Design review of the part built by this model. Coordinates are the model's own, in mm. Face numbers are marked on the shaded views. A direction names the side the tool comes from. Give positions to 0.01 mm unless a question says otherwise; leave off trailing zeros. Order: outer loops, then holes, each group sorted by start corner. A loop starts at its lowest first (then second) coordinate and runs counter-clockwise, first axis right, second up.
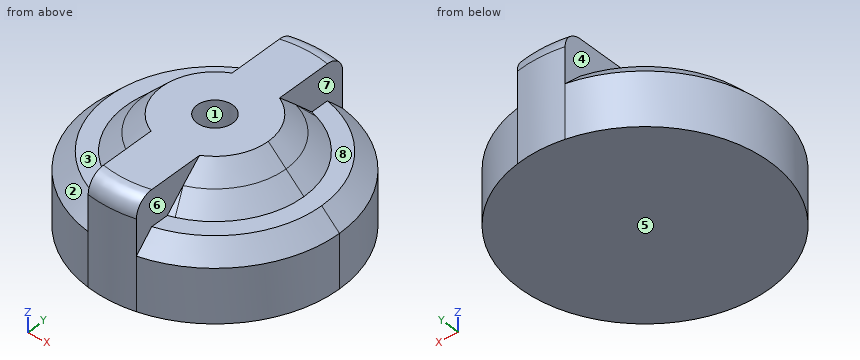
```python
from build123d import *
from build123d import SkipClean  # not in build123d's __all__

# Parameters (mm, degrees)
F0_R     = 3.175
F1_DEPTH = 12.7
F2_DEPTH = 19.05
F3_SIZE  = 3.17499
F4_DEPTH = 19.05
F5_R     = 3.175
F6_START = 6
F6_DEPTH = 15


# Not quite as in the source:
# - a fillet or chamfer is up to 0.001 mm smaller than in the source, because OpenCascade refuses the exact size


with BuildPart() as f1:
    # F0 (on Top) → F1 (new body)
    with BuildSketch(Plane.XY):
        with BuildLine():
            Line((-4.1830006975, 11.9913512652), (-4.1830006975, 21.8278063526))
            ThreePointArc((-4.1830006975, 21.8278063526), (-22.225, 0), (-4.1830006975, -21.8278063526))
            Line((-4.1830006975, -21.8278063526), (-4.1830006975, -11.9913512652))
            ThreePointArc((-4.1830006975, -11.9913512652), (-12.7, 0), (-4.1830006975, 11.9913512652))
        make_face()
        with BuildLine():
            ThreePointArc((4.3927960263, -21.7865547545), (17.1985539608, -14.0769445072), (22.225, 0))
            ThreePointArc((22.225, 0), (17.1985539608, 14.0769445072), (4.3927960263, 21.7865547545))
            Line((4.3927960263, 21.7865547545), (4.3927960263, 11.916095966))
            ThreePointArc((4.3927960263, 11.916095966), (10.4182174467, 7.2629708269), (12.7, 0))
            ThreePointArc((12.7, 0), (10.4182174467, -7.2629708269), (4.3927960263, -11.916095966))
            Line((4.3927960263, -11.916095966), (4.3927960263, -21.7865547545))
        make_face()
        with BuildLine():
            Line((4.3927960263, -11.916095966), (4.3927960263, 11.916095966))
            ThreePointArc((4.3927960263, 11.916095966), (0.1114421824, 12.6995110394), (-4.1830006975, 11.9913512652))
            Line((-4.1830006975, 11.9913512652), (-4.1830006975, -11.9913512652))
            ThreePointArc((-4.1830006975, -11.9913512652), (0.1114421824, -12.6995110394), (4.3927960263, -11.916095966))
        make_face()
        Circle(F0_R, mode=Mode.SUBTRACT)
        with BuildLine():
            Line((-4.1830006975, -11.9913512652), (-4.1830006975, 11.9913512652))
            ThreePointArc((-4.1830006975, 11.9913512652), (-12.7, 0), (-4.1830006975, -11.9913512652))
        make_face()
        with BuildLine():
            ThreePointArc((12.7, 0), (10.4182174467, 7.2629708269), (4.3927960263, 11.916095966))
            Line((4.3927960263, 11.916095966), (4.3927960263, -11.916095966))
            ThreePointArc((4.3927960263, -11.916095966), (10.4182174467, -7.2629708269), (12.7, 0))
        make_face()
        with BuildLine():
            Line((4.3927960263, 11.916095966), (4.3927960263, 21.7865547545))
            ThreePointArc((4.3927960263, 21.7865547545), (0.1069062374, 22.2247428794), (-4.1830006975, 21.8278063526))
            Line((-4.1830006975, 21.8278063526), (-4.1830006975, 11.9913512652))
            ThreePointArc((-4.1830006975, 11.9913512652), (0.1114421824, 12.6995110394), (4.3927960263, 11.916095966))
        make_face()
        with BuildLine():
            ThreePointArc((-4.1830006975, -21.8278063526), (0.1069062374, -22.2247428794), (4.3927960263, -21.7865547545))
            Line((4.3927960263, -21.7865547545), (4.3927960263, -11.916095966))
            ThreePointArc((4.3927960263, -11.916095966), (0.1114421824, -12.6995110394), (-4.1830006975, -11.9913512652))
            Line((-4.1830006975, -11.9913512652), (-4.1830006975, -21.8278063526))
        make_face()
        Circle(F0_R)
    extrude(amount=F1_DEPTH)

    # F0 (on Top) → F2 (join)
    with BuildSketch(Plane.XY):
        with BuildLine():
            ThreePointArc((12.7, 0), (10.4182174467, 7.2629708269), (4.3927960263, 11.916095966))
            Line((4.3927960263, 11.916095966), (4.3927960263, -11.916095966))
            ThreePointArc((4.3927960263, -11.916095966), (10.4182174467, -7.2629708269), (12.7, 0))
        make_face()
        with BuildLine():
            Line((-4.1830006975, -11.9913512652), (-4.1830006975, 11.9913512652))
            ThreePointArc((-4.1830006975, 11.9913512652), (-12.7, 0), (-4.1830006975, -11.9913512652))
        make_face()
        with BuildLine():
            Line((4.3927960263, -11.916095966), (4.3927960263, 11.916095966))
            ThreePointArc((4.3927960263, 11.916095966), (0.1114421824, 12.6995110394), (-4.1830006975, 11.9913512652))
            Line((-4.1830006975, 11.9913512652), (-4.1830006975, -11.9913512652))
            ThreePointArc((-4.1830006975, -11.9913512652), (0.1114421824, -12.6995110394), (4.3927960263, -11.916095966))
        make_face()
        Circle(F0_R, mode=Mode.SUBTRACT)
        Circle(F0_R)
    extrude(amount=F2_DEPTH)

    # F3 (size 3.175 in the source; OpenCascade refuses exactly that, so slightly less here)
    f3_edges = [f1.edges().sort_by_distance(p)[0] for p in [
        (4.183001, -21.827806, 12.7),
        (-4.392796, -11.916096, 12.7),
        (-4.392796, -11.916096, 19.05),
    ]]
    chamfer(f3_edges, length=F3_SIZE)

    # F0 (on Top) → F4 (join)
    with BuildSketch(Plane.XY):
        with BuildLine():
            Line((4.3927960263, 11.916095966), (4.3927960263, 21.7865547545))
            ThreePointArc((4.3927960263, 21.7865547545), (0.1069062374, 22.2247428794), (-4.1830006975, 21.8278063526))
            Line((-4.1830006975, 21.8278063526), (-4.1830006975, 11.9913512652))
            ThreePointArc((-4.1830006975, 11.9913512652), (0.1114421824, 12.6995110394), (4.3927960263, 11.916095966))
        make_face()
        with BuildLine():
            Line((4.3927960263, -11.916095966), (4.3927960263, 11.916095966))
            ThreePointArc((4.3927960263, 11.916095966), (0.1114421824, 12.6995110394), (-4.1830006975, 11.9913512652))
            Line((-4.1830006975, 11.9913512652), (-4.1830006975, -11.9913512652))
            ThreePointArc((-4.1830006975, -11.9913512652), (0.1114421824, -12.6995110394), (4.3927960263, -11.916095966))
        make_face()
        Circle(F0_R, mode=Mode.SUBTRACT)
        with BuildLine():
            ThreePointArc((-4.1830006975, -21.8278063526), (0.1069062374, -22.2247428794), (4.3927960263, -21.7865547545))
            Line((4.3927960263, -21.7865547545), (4.3927960263, -11.916095966))
            ThreePointArc((4.3927960263, -11.916095966), (0.1114421824, -12.6995110394), (-4.1830006975, -11.9913512652))
            Line((-4.1830006975, -11.9913512652), (-4.1830006975, -21.8278063526))
        make_face()
    with SkipClean():  # cleaning this boolean's faces spoils the solid; the shape is the same uncleaned
        extrude(amount=F4_DEPTH)

    # F5
    f5_edges = [f1.edges().sort_by_distance(p)[0] for p in [
        (0.106906, -22.224743, 19.05),
        (0.106906, 22.224743, 19.05),
    ]]
    fillet(f5_edges, radius=F5_R)

    # F0 (on Top) → F6 (cut)
    with BuildSketch(Plane.XY.offset(F6_START)):
        Circle(F0_R)
    extrude(amount=F6_DEPTH, mode=Mode.SUBTRACT)


solid = f1.part
```
1. Take a section at A-A (z = 5). State the section outline as (x, y) points (3 decimals), then the cut area to 3 significant figures.
Recorded:
outline: circle Ø44.45 at (0, 0)
area: 1,550 mm2
2. For pin 1 (5 mm diameter, centred on y = -18, z = 15.5, fed in from -X); pin 2 (1 mm diameter, centred on x = 8, z = 7.5, fed in from -Y); pin 3 (4 mm diameter, centred on y = 6.5, z = 9, fed in from -X), all flat-tipped, find the tip position at first contact; note any pin that passes through.
Recorded:
pin 1: stops at x = -4.18
pin 2: stops at y = -20.92
pin 3: stops at x = -21.76
3. For line 1 along Y through (x, z) = (0, 12.25) (3 decimals); line 2 along X through (y, z) = (0, 10.75) (3 decimals); line 3 along Y through (x, z) = (0.5, 11.75), list the stretches that pass through material, from the lowest coordinate up.
Recorded:
line 1: y = -22.225 to -3.175, 3.175 to 22.225
line 2: x = -21 to -3.175, 3.175 to 21
line 3: y = -22.22 to -3.14, 3.14 to 22.22
4. Draft analysis for pull direction Y (two halves, no side actions). For the marked faces 1, 2 and 3, state which applies: pulls with the +Y half, pulls with the -Y half, needs draft (parallel to the pull), parting line crosses it, or undercut.
Recorded:
face 1: undercut
face 2: parting line crosses it
face 3: needs draft
5. Machinability: for the marked faces 4, 5, 6, 7 and 8, which of the approach directions +Z, -Z, +X, -X, +Y, -Y give a long, thin tool a straight path to every point of the face, cutting with its end or side? Answer none if there is none.
Recorded:
face 4: +Z, -X, +Y
face 5: -Z, +X, -X, +Y, -Y
face 6: +Z, +X, -Y
face 7: +Z, +X, +Y
face 8: +Z, +X
